Can you work these out from the model? Positions are in its coordinate system, mm. Face numbers are marked on the shaded views. A direction names the side the tool comes from. Give positions to 0.01 mm unless a question says otherwise; leave off trailing zeros. Order: outer loops, then holes, each group sorted by start corner. A loop starts at its lowest first (then second) coordinate and runs counter-clockwise, first axis right, second up. Notation, with made-up numbers: M -4,-3 L 35,-3 A10 cw 35,14 Z; hole C 6,-19.5 d10. An arc over 180 degrees is marked long. Answer as a JSON object with one key per item and string values.
Autodesk Inventor part; units mm, degrees
ref_plane "YZ Plane" through (0, 0, 0) normal (1, 0, 0) x (0, 1, 0)
ref_plane "XZ Plane" through (0, 0, 0) normal (0, 1, 0) x (-1, 0, 0)
ref_plane "XY Plane" through (0, 0, 0) normal (0, 0, 1) x (1, 0, 0)
sketch "Sketch8" plane through (0, 0, 0) normal (0, 1, 0) x (-1, 0, 0)
  line L0 (-61, -56) -> (61, -56)
  line L1 (61, -56) -> (61, 56)
  line L2 (61, 56) -> (-61, 56)
  line L3 (-61, 56) -> (-61, -56)
  line L4 (-61, -56) -> (61, 56) construction
  line L5 (61, -56) -> (-61, 56) construction
  point P0 (0, 0)
  dimension "d26" = 122
  dimension "d27" = 112
extrude "Extrusion7" add sketch "Sketch8" along normal blind 95
sketch "Sketch9" plane through (0, 0, 0) normal (0, -1, 0) x (1, 0, 0)
  line L0 (-61, 56) -> (61, 56)
  line L1 (-61, -56) -> (61, -56)
  line L2 (61, -56) -> (61, 56)
  line L3 (61, 56) -> (-61, 56)
  line L4 (-61, 56) -> (-61, -56)
  line L5 (-61, -56) -> (61, 56) construction
  line L6 (61, -56) -> (-61, 56) construction
  line L7 (57, 52) -> (57, -52)
  line L8 (57, -52) -> (-61, -52)
  line L9 (-61, 52) -> (57, 52)
  line L10 (53, -48) -> (53, 48)
  line L11 (53, 48) -> (-61, 48)
  line L12 (-61, -48) -> (53, -48)
  line L13 (-58.8844, -52) -> (-58.8844, -54.0578)
  line L14 (-58.8844, 54.0578) -> (-58.8844, 52)
  line L15 (-54.6854, 48) -> (-54.6854, 50.203)
  line L16 (-54.6854, -50.203) -> (-54.6854, -48)
  point P0 (0, 0)
  dimension "d30" = 4
  dimension "d31" = 4
  dimension "d47" = 4
  dimension "d48" = 4
  dimension "d49" = 4
  dimension "d50" = 4
extrude "Extrusion8" cut sketch "Sketch9" against normal blind 115 contours L11 L10 L12 L4
extrude "Extrusion9" cut sketch "Sketch9" against normal blind 90 contours L9 L7 L8 L4 L12 L10 L11
sketch "Sketch10" plane through (0, 0, 0) normal (0, -1, 0) x (1, 0, 0)
  line L0 (61, -56) -> (-61, -56)
  line L1 (-61, -56) -> (-61, 56)
  line L2 (-61, 56) -> (61, 56)
  line L3 (61, 56) -> (61, -56)
  line L4 (61, -56) -> (-61, 56) construction
  line L5 (-61, -56) -> (61, 56) construction
  line L6 (-65, 60) -> (-65, -60)
  line L7 (-65, -60) -> (65, -60)
  line L8 (65, -60) -> (65, 60)
  line L9 (65, 60) -> (-65, 60)
  line L10 (-61, 56) -> (-65, 56)
  line L11 (-61, -56) -> (-65, -56)
  line L12 (-61, 56) -> (-61, 60)
  line L13 (-61, -56) -> (-61, -60)
  point P0 (0, 0)
  dimension "d36" = 4
extrude "Extrusion10" add sketch "Sketch10" against normal blind 5 contours L3 L2 L12 L9 L8 L7 L13 L0
sketch "Sketch11" plane through (0, 0, 0) normal (0, -1, 0) x (1, 0, 0)
  circle A0 centre (-71, 9) radius 135
  line L0 (57, 52) -> (57, -52)
  line L1 (65, -60) -> (65, 60)
  circle A1 centre (-71, 9) radius 110
  line L2 (14.668, -60) -> (65, -60)
  line L3 (65, -60) -> (65, 60)
  line L4 (65, 60) -> (26.4628, 60)
  line L5 (-61, 60) -> (65, 60)
  point P0 (0, 0)
  dimension "d39" = 270
  dimension "d41" = 136
  dimension "d42" = 220
extrude "Extrusion11" cut sketch "Sketch11" against normal blind 1.125 contours A0 L0 | A0 L4 L1 L2 | L0 A0 L2 A1 L4
properties part number "Galvo Housing-01"
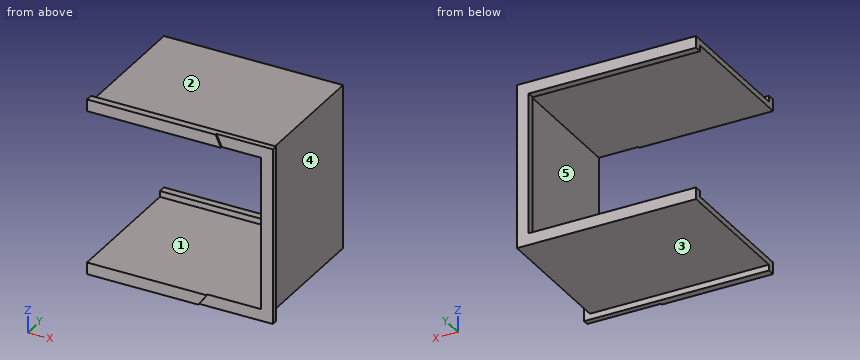
1) Thinking about a two-plate mould opening in Z: for the marked faces 3, 4 and 5, which applies, pulls with the +Z half, pulls with the -Z half, needs draft (parallel to the pull), parting line crosses it, or undercut?
Results found:
{"face 3": "pulls with the -Z half", "face 4": "needs draft", "face 5": "undercut"}
2) I'm going to push flat-ended pins straight in: pin 1 Ø5 at (x, y) = (-5, 55) entering from +Z; pin 2 Ø5 at (x, y) = (-32, 38) entering from -Z; pin 3 Ø5 at (y, z) = (79.5, 38.5) entering from -X. Where does each tip first touch, or does it pass through?
Results found:
{"pin 1": "stops at z = 56", "pin 2": "stops at z = -56", "pin 3": "stops at x = 57"}
3) I need wall thicknesses on L1, parallel to Z at x = 8, y = 22; L2, parallel to Z at x = 12, y = 91.5; L3, parallel to X at y = 62.5, z = 22. Which ranges of each line are inside material? Lowest first, please.
Results found:
{"L1": "z = -56 to -52, 52 to 56", "L2": "z = -56 to -48, 48 to 56", "L3": "x = 57 to 61"}
4) For the marked faces 1 and 2, which set-ups out of +Z, -Z, +X, -X, +Y, -Y let a thin tool reach every point of the face, with its end or its side?
Results found:
{"face 1": "-X, -Y", "face 2": "+Z, +X, -X, +Y"}
5) I want a section at B-B on y = 49.5. Write out the boundary of the cut face in (x, z), and give its area (3 significant figures).
Results found:
{"outline": "M -61,-56 L 61,-56 L 61,56 L -61,56 L -61,52 L 57,52 L 57,-52 L -61,-52 Z", "area": "1,390 mm²"}
6) I want a section at C-C on z = 13.5. Write out the boundary of the cut face in (x, y) (3 decimals), and give its area (3 significant figures).
Results found:
{"outline": "M 53,90 L 57,90 L 57,1.125 L 65,1.125 L 65,5 L 61,5 L 61,95 L 53,95 Z", "area": "411 mm²"}
7) I want a section at A-A on x = 0. Write out the boundary of the cut face in (y, z).
Results found:
{"outline": "M 0,-60 L 5,-60 L 5,-56 L 95,-56 L 95,-48 L 90,-48 L 90,-52 L 0,-52 Z; M 0,52 L 90,52 L 90,48 L 95,48 L 95,56 L 5,56 L 5,60 L 0,60 Z"}
